```python
from build123d import *

# Parameters (mm, degrees)
F1_DEPTH = 55
F3_DEPTH = 32.001
F4_R     = 5
F5_R     = 5
F7_DEPTH = 20
F9_DEPTH = 6


# Not quite as in the source:
# - a feature names something its author has since deleted; it is built from what else it names


with BuildPart() as f1:
    # F0 (on Front) → F1 (new body)
    with BuildSketch(Plane.XZ):
        Polygon((0, 35), (0, 0), (38, 0), (38, 47.5), (23, 47.5), (17, 32), (11, 32), (11, 35), align=None)
    extrude(amount=F1_DEPTH)

    # F2 (on face) → F3 (cut, through all)
    with BuildSketch(Plane.XY.offset(32)):
        with BuildLine():
            ThreePointArc((14, -5), (11.8786796564, -5.8786796564), (11, -8))
            Line((11, -8), (11, -14.5))
            ThreePointArc((11, -14.5), (11.8786796564, -16.6213203436), (14, -17.5))
            ThreePointArc((14, -17.5), (16.1213203436, -16.6213203436), (17, -14.5))
            Line((17, -14.5), (17, -8))
            ThreePointArc((17, -8), (16.1213203436, -5.8786796564), (14, -5))
        make_face()
        with BuildLine():
            ThreePointArc((14, -37.5), (11.8786796564, -38.3786796564), (11, -40.5))
            Line((11, -40.5), (11, -47))
            ThreePointArc((11, -47), (11.8786796564, -49.1213203436), (14, -50))
            ThreePointArc((14, -50), (16.1213203436, -49.1213203436), (17, -47))
            Line((17, -47), (17, -40.5))
            ThreePointArc((17, -40.5), (16.1213203436, -38.3786796564), (14, -37.5))
        make_face()
    extrude(amount=-F3_DEPTH, mode=Mode.SUBTRACT)

    # F4
    f4_edges = [f1.edges().sort_by_distance(p)[0] for p in [
        (38, -55, 23.75),
        (38, 0, 23.75),
    ]]
    fillet(f4_edges, radius=F4_R)

    # F5
    f5_edges = [f1.edges().sort_by_distance(p)[0] for p in [
        (0, 0, 17.5),
        (0, -55, 17.5),
    ]]
    fillet(f5_edges, radius=F5_R)

    # F6 (on face) → F7 (cut)
    with BuildSketch(Plane(origin=(0, 0, 0), x_dir=(1, 0, 0), z_dir=(0, 0, -1))):
        with BuildLine():
            Line((27, 52), (7, 52))
            ThreePointArc((7, 52), (3.4644660941, 50.5355339059), (2, 47))
            Line((2, 47), (2, 8))
            ThreePointArc((2, 8), (3.4644660941, 4.4644660941), (7, 3))
            Line((7, 3), (27, 3))
            ThreePointArc((27, 3), (30.5355339059, 4.4644660941), (32, 8))
            Line((32, 8), (32, 47))
            ThreePointArc((32, 47), (30.5355339059, 50.5355339059), (27, 52))
        make_face()
        with BuildLine():
            ThreePointArc((17, 8), (14, 5), (11, 8))
            Line((11, 8), (11, 14.5))
            ThreePointArc((11, 14.5), (14, 17.5), (17, 14.5))
            Line((17, 14.5), (17, 8))
        make_face(mode=Mode.SUBTRACT)
        with BuildLine():
            Line((17, 47), (17, 40.5))
            ThreePointArc((17, 40.5), (14, 37.5), (11, 40.5))
            Line((11, 40.5), (11, 47))
            ThreePointArc((11, 47), (14, 50), (17, 47))
        make_face(mode=Mode.SUBTRACT)
    extrude(amount=-F7_DEPTH, mode=Mode.SUBTRACT)

    # F8 (on face) → F9 (cut)
    with BuildSketch(Plane.YZ.offset(38)):
        with BuildLine():
            Line((-47.75, 0), (-39.75, 0))
            ThreePointArc((-39.75, 0), (-43.75, 4), (-47.75, 0))
        make_face()
        with BuildLine():
            ThreePointArc((-7.25, 0), (-11.25, 4), (-15.25, 0))
            Line((-15.25, 0), (-7.25, 0))
        make_face()
    extrude(amount=-F9_DEPTH, mode=Mode.SUBTRACT)


solid = f1.part
```
Input: part model. Units: mm. Frame: model coordinates. A direction names the side the tool comes from. Coordinates: 2 decimals unless noted, no trailing zeros. Loops run counter-clockwise (first coordinate to the right, second up) from the corner with the lowest first, then second, coordinate; pieces in that order, holes last. Notation, with made-up numbers: M 83.5,30 L 135.5,30 A25 cw 135.5,46 Z; hole C 3.25,5 d5. An arc over 180 degrees is marked long. One line per item, written item: value.
(1) Section B-B (y = -43.75). Output: boundary loops of the cut face in (x, z), and give its area (3 significant figures).
Filled in:
outline: M 0,0 L 2,0 L 2,20 L 11,20 L 11,35 L 0,35 Z; M 17,20 L 32,20 L 32,4 L 38,4 L 38,47.5 L 23,47.5 L 17,32 Z
area: 832 mm^2
(2) Pull-direction query (Y, two-part tool) for faces 1 (the flat face through (35, -27, 0)), 2 (the flat face through (32, -27, 10)); classes: +Y half, -Y half, draft (parallel to the pull), parting line (faces both ways), or undercut.
Filled in:
face 1: draft
face 2: undercut
(3) Line query: line 1 along Y through (x, z) = (14, 25); line 2 along X through (y, z) = (-22.5, 17); line 3 along Y through (x, z) = (9, 17). Output: solid intervals per line, ascending. Write a range as from..to.
Filled in:
line 1: -55..-50, -37.5..-17.5, -5..0
line 2: 0..2, 32..38
line 3: -55..-52, -3..0
(4) Pin query (flat end, axial travel): pin 1 (1.8 mm diameter, centred on x = 14, y = -29.5, fed in from +Z); pin 2 (1.5 mm diameter, centred on x = 31.5, y = -46, fed in from -Z); pin 3 (8 mm diameter, centred on x = 6.5, y = -39.5, fed in from -Z). Return the tip coordinate at first contact, or that it passes through.
Filled in:
pin 1: z = 32
pin 2: z = 2.85
pin 3: z = 20
(5) Reachability of faces 3 (the cylindrical face through (35, -43.7, 4)), 4 (the flat face through (17, -28, 20)), 5 (the flat face through (6, -27, 35)), 6 (the flat face through (17, -11, 26)) from +Z, -Z, +X, -X, +Y, -Y: full face, straight path, thin tool, end or side. Return the list, or none.
Filled in:
face 3: -Z, +X
face 4: -Z
face 5: +Z, -X, +Y, -Y
face 6: +Z, -Z
(6) Section C-C (x = 25.5). Output: boundary loops of the cut face in (y, z).
Filled in:
outline: M -55,0 L -52,0 L -52,20 L -3,20 L -3,0 L 0,0 L 0,47.5 L -55,47.5 Z
(7) Section A-A (z = 9.5). Output: boundary loops of the cut face in (x, y), and give its area (3 significant figures).
Filled in:
outline: M 0,-50 A5 ccw 5,-55 L 33,-55 A5 ccw 38,-50 L 38,-5 A5 ccw 33,0 L 5,0 A5 ccw 0,-5 Z; hole M 2,-47 A5 ccw 7,-52 L 27,-52 A5 ccw 32,-47 L 32,-8 A5 ccw 27,-3 L 7,-3 A5 ccw 2,-8 Z
area: 620 mm^2
(8) Section D-D (y = -29). Output: boundary loops of the cut face in (x, z), and give its area (3 significant figures).
Filled in:
outline: M 0,0 L 2,0 L 2,20 L 32,20 L 32,0 L 38,0 L 38,47.5 L 23,47.5 L 17,32 L 11,32 L 11,35 L 0,35 Z
area: 928 mm^2
